```python
from build123d import *

# Parameters (mm, degrees)
F0_R     = 6.45
F1_DEPTH = 1.2


with BuildPart() as f1:
    # F0 (on Top) → F1 (new body)
    with BuildSketch(Plane.XY):
        with BuildLine():
            Line((0.55, -14.300229), (0.55, -7.640229))
            ThreePointArc((0.55, -7.640229), (0, 7.66), (-0.55, -7.640229))
            Line((-0.55, -7.640229), (-0.55, -14.300229))
            Line((-0.55, -14.300229), (-4.229019, -14.300229))
            Line((-4.229019, -14.300229), (-4.229019, -15.400229))
            Line((-4.229019, -15.400229), (-0.55, -15.400229))
            Line((-0.55, -15.400229), (-0.55, -20.640229))
            Line((-0.55, -20.640229), (0.55, -20.640229))
            Line((0.55, -20.640229), (0.55, -15.400229))
            Line((0.55, -15.400229), (4.229019, -15.400229))
            Line((4.229019, -15.400229), (4.229019, -14.300229))
            Line((4.229019, -14.300229), (0.55, -14.300229))
        make_face()
        Circle(F0_R, mode=Mode.SUBTRACT)
    extrude(amount=F1_DEPTH)


solid = f1.part
```
Can you work these out from the model? Positions are in its coordinate system, mm. A direction names the side the tool comes from. Coordinates: 2 decimals unless noted, no trailing zeros. Loops run counter-clockwise (first coordinate to the right, second up) from the corner with the lowest first, then second, coordinate; pieces in that order, holes last. Notation, with made-up numbers: (-40, 6.5) -> (16, 6.5) arc R21 ccw to (16, 10.5) -> close; hole circle Ø6 at (81.25, 4.5). An arc over 180 degrees is marked (long way). Put each result on its own line as item: value. Start each with the question number.
Q1. Thinking about a two-plate mould opening in Y: for faces 4 (the face through (2, -15.4, 1)), 5 (the face through (0.55, -11, 1)), 6 (the face through (-0.55, -18, 1)), which applies, pulls with the +Y half, pulls with the -Y half, needs draft (parallel to the pull), parting line crosses it, or undercut?
Q2. For faces 1 (the face through (2, -14.3, 1)), 2 (the face through (-2, -14.3, 1)), 3 (the face through (0.55, -18, 1)), which set-ups out of +Z, -Z, +X, -X, +Y, -Y let a thin tool reach every point of the face, with its end or its side?
Q3. If I drill on line 1 (Y direction, x = 0, z = 0.9); line 2 (Y direction, x = -4, z = 1); line 3 (Y direction, x = -3, z = 0.95), over which ranges is the centre line in solid material (lowest first)? Write a range as [from, to].
Q4. I want a section at A-A (y = 0). Write out the boundary of the cut face in (x, z).
Q5. I want a section at D-D (x = -2). Write out the boundary of the cut face in (y, z), plus the area to 3 significant figures.
Q6. I'm going to push flat-ended pins straight in: P1, Ø8, axis at x = -3, y = -3, coming from the +Z side; P2, Ø0.6, axis at x = -3, z = 0.5, coming from the +Y side; P3, Ø0.6, axis at y = -19, z = 1, coming from the +X side. Where does each tip first touch, or does it pass through?
Q7. I want a section at C-C (x = 0). Write out the boundary of the cut face in (y, z).
Q8. I want a section at B-B (z = 0.4). Write out the boundary of the cut face in (x, y), plus the area to 3 significant figures.
Taken from the geometry:
1. face 4: pulls with the -Y half
1. face 5: undercut
1. face 6: needs draft
2. face 1: +Z, -Z, +X
2. face 2: +Z, -Z, -X
2. face 3: +Z, -Z, +X, -Y
3. line 1: y = [-20.64, -6.45], [6.45, 7.66]
3. line 2: y = [-15.4, -14.3], [-6.53, -5.06], [5.06, 6.53]
3. line 3: y = [-15.4, -14.3], [-7.05, -5.71], [5.71, 7.05]
4. outline: (-7.66, 0) -> (-6.45, 0) -> (-6.45, 1.2) -> (-7.66, 1.2) -> close; (6.45, 0) -> (7.66, 0) -> (7.66, 1.2) -> (6.45, 1.2) -> close
5. outline: (-15.4, 0) -> (-14.3, 0) -> (-14.3, 1.2) -> (-15.4, 1.2) -> close; (-7.39, 0) -> (-6.13, 0) -> (-6.13, 1.2) -> (-7.39, 1.2) -> close; (6.13, 0) -> (7.39, 0) -> (7.39, 1.2) -> (6.13, 1.2) -> close
5. area: 4.35 mm2
6. P1: stops at z = 1.2
6. P2: stops at y = 7.17
6. P3: stops at x = 0.55
7. outline: (-20.64, 0) -> (-6.45, 0) -> (-6.45, 1.2) -> (-20.64, 1.2) -> close; (6.45, 0) -> (7.66, 0) -> (7.66, 1.2) -> (6.45, 1.2) -> close
8. outline: (-4.23, -15.4) -> (-0.55, -15.4) -> (-0.55, -20.64) -> (0.55, -20.64) -> (0.55, -15.4) -> (4.23, -15.4) -> (4.23, -14.3) -> (0.55, -14.3) -> (0.55, -7.64) arc R7.66 ccw (long way) to (-0.55, -7.64) -> (-0.55, -14.3) -> (-4.23, -14.3) -> close; hole circle Ø12.9 at (0, 0)
8. area: 76.0 mm2
